Autodesk Inventor part; units mm, degrees
ref_plane "YZ Plane" through (0, 0, 0) normal (1, 0, 0) x (0, 1, 0)
ref_plane "XZ Plane" through (0, 0, 0) normal (0, 1, 0) x (-1, 0, 0)
ref_plane "XY Plane" through (0, 0, 0) normal (0, 0, 1) x (1, 0, 0)
sketch "Sketch1" plane through (0, 0, 0) normal (0, 0, 1) x (1, 0, 0)
  circle A0 centre (0, 0) radius 9.525
  line L0 (0, 0) -> (0, 6.35) construction
  line L1 (3.6695, 6.35) -> (7.334, -0.0028)
  line L2 (7.334, -0.0028) -> (3.6645, -6.3528)
  line L3 (3.6645, -6.3528) -> (-3.6695, -6.35)
  line L4 (-3.6695, -6.35) -> (-7.334, 0.0028)
  line L5 (-7.334, 0.0028) -> (-3.6645, 6.3528)
  line L6 (-3.6645, 6.3528) -> (3.6695, 6.35)
  dimension "d0" = 19.05
  dimension "d1" = 6.35
extrude "Extrusion1" add sketch "Sketch1" along normal blind 3.302
properties part number "3D Model Spacer Arm"
Read the model definition and answer for the solid it produces. Units are mm, in the model's axes. A direction names the side the tool comes from. Round coordinates to 2 decimals unless told otherwise and drop trailing zeros. Write each loop counter-clockwise with the first axis right and the second up, starting at its lowest first coordinate (ties: lowest second). Pieces come first, ordered by that corner, then holes. Notation, with made-up numbers: M -15.5,63.25 L 7.5,63.25 A20 cw 7.5,67.25 Z; hole C 0,80 d9. An arc over 180 degrees is marked long. Use a Markdown table: item, result.
1) For a pull along X with two mould halves and no side action, classify faces 3 (the flat face through (5.476, 3.218, 1.628)), 4 (the flat face through (6.2, 2.3, 0)), 5 (the cylindrical face through (-7.559, 5.796, 1.628)) as pulls with the +X half, pulls with the -X half, needs draft (parallel to the pull), parting line crosses it, or undercut.
Answers follow:
| item | result |
|---|---|
| face 3 | undercut |
| face 4 | needs draft |
| face 5 | parting line crosses it |
2) The part is cut by section B-B (x = 0). Write down the section's boundary in (y, z) (3 decimals), plus the area to 3 significant figures.
Answers follow:
| item | result |
|---|---|
| outline | M -9.525,0 L -6.351,0 L -6.351,3.302 L -9.525,3.302 Z; M 6.351,0 L 9.525,0 L 9.525,3.302 L 6.351,3.302 Z |
| area | 21.0 mm2 |
3) A tool of negligible diameter and unlimited length cuts with its end or side. For faces 1 (the flat face through (6.2, 2.3, 3.302)), 2 (the flat face through (-5.525, 3.133, 1.628)), from which of +Z, -Z, +X, -X, +Y, -Y can it reach the whole face along a straight path? Write none if from no direction.
Answers follow:
| item | result |
|---|---|
| face 1 | +Z, +X, -X, +Y, -Y |
| face 2 | +Z, -Z |
4) The part is cut by section C-C (y = -3). Write down the section's boundary in (x, z), plus the area to 3 significant figures.
Answers follow:
| item | result |
|---|---|
| outline | M -9.04,0 L -5.6,0 L -5.6,3.3 L -9.04,3.3 Z; M 5.6,0 L 9.04,0 L 9.04,3.3 L 5.6,3.3 Z |
| area | 22.7 mm2 |
5) Straight lines are drawn through the part: line 1 along Y through (x, z) = (0, 3) (3 decimals); line 2 along Y through (x, z) = (6, 1.25); line 3 along X through (y, z) = (-6.25, 1.2). For each, find the intervals that lie inside material, in ascending order. Write a range as [from, to].
Answers follow:
| item | result |
|---|---|
| line 1 | y = [-9.525, -6.351], [6.351, 9.525] |
| line 2 | y = [-7.4, -2.31], [2.31, 7.4] |
| line 3 | x = [-7.19, -3.73], [3.72, 7.19] |
